Here's the drawing with two shaded views (mm, measured from the low corner). I have some questions. A direction names the side the tool comes from. Give positions to 0.01 mm unless a question says otherwise; leave off trailing zeros. Order: outer loops, then holes, each group sorted by start corner. A loop starts at its lowest first (then second) coordinate and runs counter-clockwise, first axis right, second up. Notation, with made-up numbers: M 45.25,17.25 L 84.25,17.25 A19 ccw 84.25,51.25 Z; hole C -8.75,67 d11. An arc over 180 degrees is marked long. Write each question's results on one line, items separated by ' | '.
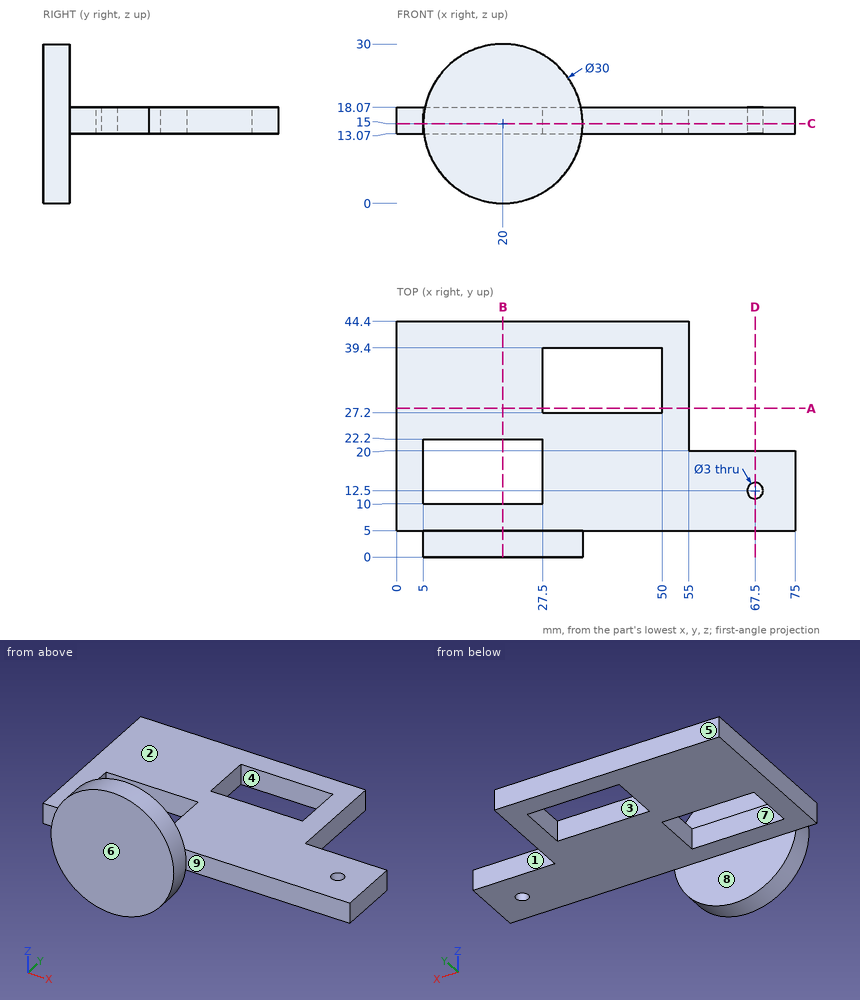
(1) For the marked faces 5, 6, 7, 8 and 9, which set-ups out of +Z, -Z, +X, -X, +Y, -Y let a thin tool reach every point of the face, with its end or its side?
Data:
face 5: +Z, -Z, +X, -X, +Y | face 6: +Z, -Z, +X, -X, -Y | face 7: +Z, -Z | face 8: -Z, +X, -X, +Y | face 9: +Z, -Z, +X, -Y
(2) Imagine slicing it at B-B, the plane x = 20. Write out the boundary of the cut face in (y, z), plus the area to 3 significant figures.
Data:
outline: M 0,0 L 5,0 L 5,13.07 L 10,13.07 L 10,18.07 L 5,18.07 L 5,30 L 0,30 Z; M 22.2,13.07 L 44.4,13.07 L 44.4,18.07 L 22.2,18.07 Z | area: 286 mm2
(3) Will these pins go through, and if not, where does the flat tip stop? P1, Ø4, axis at x = 35, z = 15.5, coming from the -Y side; P2, Ø1.5, axis at x = 12, z = 22, coming from the +Y side; P3, Ø5, axis at x = 67.5, y = 12.5, coming from the +Z side; P4, Ø4, axis at y = 33, z = 15, coming from the +X side.
Data:
P1: stops at y = 0 | P2: stops at y = 5 | P3: stops at z = 18.07 | P4: stops at x = 55
(4) Imagine slicing it at D-D, the plane x = 67.5. Write out the boundary of the cut face in (y, z).
Data:
outline: M 5,13.07 L 11,13.07 L 11,18.07 L 5,18.07 Z; M 14,13.07 L 20,13.07 L 20,18.07 L 14,18.07 Z
(5) Imagine slicing it at C-C, the plane z = 15. Write out the boundary of the cut face in (x, y), plus the area to 3 significant figures.
Data:
outline: M 0,5 L 5,5 L 5,0 L 35,0 L 35,5 L 75,5 L 75,20 L 55,20 L 55,44.4 L 0,44.4 Z; hole M 5,10 L 27.5,10 L 27.5,22.2 L 5,22.2 Z; hole M 27.5,27.2 L 50,27.2 L 50,39.4 L 27.5,39.4 Z; hole C 67.5,12.5 d3 | area: 2,060 mm2
(6) We'd pull the mould along Y, two halves only. Please class the marked faces 1, 2, 3 and 4: +Y half, -Y half, draft (parallel to the pull), parting line (faces both ways), or undercut.
Data:
face 1: +Y half | face 2: draft | face 3: undercut | face 4: undercut
(7) Imagine slicing it at A-A, the plane y = 28. Write out the boundary of the cut face in (x, z).
Data:
outline: M 0,13.07 L 27.5,13.07 L 27.5,18.07 L 0,18.07 Z; M 50,13.07 L 55,13.07 L 55,18.07 L 50,18.07 Z
(8) I need wall thicknesses on L1, parallel to Y at x = 67.5, z = 16.55; L2, parallel to Z at x = 38, y = 25; L3, parallel to Y at x = 26.5, z = 22.75. Which ranges of each line are inside material? Lowest first, please. Write a range as from..to.
Data:
L1: y = 5..11, 14..20 | L2: z = 13.07..18.07 | L3: y = 0..5
